Geometry check sheet. Reference: the model listing, model coordinates, mm. A direction names the side the tool comes from. Round coordinates to 2 decimals unless told otherwise and drop trailing zeros. Write each loop counter-clockwise with the first axis right and the second up, starting at its lowest first coordinate (ties: lowest second). Pieces come first, ordered by that corner, then holes.
Item 1: Cross-section at C-C (x = 24). Enter the section's corners in (y, z), then the cut area to 3 significant figures.
Item 2: Cross-section at B-B (y = 42). Enter the section's corners in (x, z).
Item 3: Access from +Z, -Z, +X, -X, +Y, -Y to the whole of each face (thin tool, end or side, straight path). Record for faces 1 (the face through (2, 8, 9.44)), 2 (the face through (6.27, 1.163, 4.689)), 3 (the face through (-0.5, 41, 4)), 4 (the face through (-0.5, 33, 10)).
Item 4: Cross-section at A-A (z = 8.75). Enter the section's corners in (x, y).
Item 5: Draft check along Y on faces 5 (the face through (6.27, 51.3, 4.63)), 6 (the face through (38.4, 26, 4)), 7 (the face through (18.04, 3.65, 1.27)), 8 (the face through (-1.57, 4.15, 0.11)). Enter one of: pulls with the +Y half, pulls with the -Y half, needs draft (parallel to the pull), parting line crosses it, or undercut.
Item 6: Cross-section at D-D (x = 34). Enter the section's corners in (y, z), then the cut area to 3 significant figures.
Item 7: Scan lines: probe 1 along Y at (x, z) = (16, 3); probe 2 along X at (y, z) = (20, 2.5); probe 3 along X at (y, z) = (44.5, 5.5). Record each from-to range of solid material in increasing order.
Item 8: Depth check by flat-ended pin: P1, Ø8, axis at x = 30.5, y = 36.5, coming from the -Z side; P2, Ø2, axis at x = 28, z = 4.5, coming from the +Y side; P3, Ø0.8, axis at y = 32, z = 11, coming from the +X side; P4, Ø1, axis at x = 2, y = 45, coming from the +Z side. Enter the tip coordinate at first touch or a pass-through.
from build123d import *

# Parameters (mm, degrees)
SKETCH003_R     = 0.75
PAD002_DEPTH    = 40.4
SKETCH002_W     = 37.4
SKETCH002_H     = 43
POCKET_DEPTH    = 13
SKETCH004_W     = 9
SKETCH004_H     = 3.2
POCKET001_DEPTH = 2
POCKET005_DEPTH = 2
POCKET006_DEPTH = 2
SKETCH015_W     = 46
SKETCH015_H     = 40.4
POCKET010_DEPTH = 2.5
SKETCH018_W     = 3.6
SKETCH018_H     = 1.8
SKETCH018_W_2   = 10
SKETCH018_W_3   = 3
PAD004_DEPTH    = 10.5
SKETCH020_W     = 38.2
SKETCH020_H     = 33.9
POCKET013_DEPTH = 2.6
POCKET015_DEPTH = 23.5
FILLET004_R     = 1.5
FILLET005_R     = 0.6
FILLET006_R     = 1.35


with BuildPart() as part:
    # Sketch003 → Pad002 (new body)
    with BuildSketch(Plane(origin=(-2, 0, 0), x_dir=(0, -1, 0), z_dir=(-1, 0, 0))):
        with BuildLine():
            Line((-3.2, 6), (1.170226, 1.888902))
            ThreePointArc((-2.940872, -2.481324), (1.29979, -2.35176), (1.170226, 1.888902))
            Line((-5.578597, 0), (-2.940872, -2.481324))
            Line((-5.578597, 0), (-46.821403, 0))
            Line((-46.821403, 0), (-49.459128, -2.481324))
            ThreePointArc((-53.570226, 1.888902), (-53.69979, -2.35176), (-49.459128, -2.481324))
            Line((-49.2, 6), (-53.570226, 1.888902))
            Line((-49.2, 9), (-49.2, 6))
            Line((-3.2, 9), (-49.2, 9))
            Line((-3.2, 9), (-3.2, 6))
        make_face()
        with Locations((-51.514677, -0.296211)):
            Circle(SKETCH003_R, mode=Mode.SUBTRACT)
        with Locations((-0.885323, -0.296211)):
            Circle(SKETCH003_R, mode=Mode.SUBTRACT)
    extrude(amount=-PAD002_DEPTH)

    # Sketch002 → Pocket (cut)
    with BuildSketch(Plane(origin=(0, 0, 0.7), x_dir=(-1, 0, 0), z_dir=(0, 0, -1))):
        with Locations((-18.2, 26.2)):
            Rectangle(SKETCH002_W, SKETCH002_H)
    extrude(amount=-POCKET_DEPTH, mode=Mode.SUBTRACT)

    # Sketch004 (on Face4 of Pocket) → Pocket001 (cut)
    with BuildSketch(Plane(origin=(-2, 0, 0), x_dir=(0, -1, 0), z_dir=(-1, 0, 0))):
        with Locations((-26.4, 5.93)):
            Rectangle(SKETCH004_W, SKETCH004_H)
    extrude(amount=-POCKET001_DEPTH, mode=Mode.SUBTRACT)

    # Sketch010 (on Face5 of Pocket001) → Pocket005 (cut)
    with BuildSketch(Plane.YZ.offset(38.4)):
        with BuildLine():
            ThreePointArc((7.8, 9.05), (6.4, 7.65), (7.8, 6.25))
            Line((7.8, 6.25), (12.8, 6.25))
            ThreePointArc((12.8, 6.25), (14.2, 7.65), (12.8, 9.05))
            Line((12.8, 9.05), (7.8, 9.05))
        make_face()
        with BuildLine():
            ThreePointArc((39.6, 9.05), (38.2, 7.65), (39.6, 6.25))
            Line((39.6, 6.25), (44.6, 6.25))
            ThreePointArc((44.6, 6.25), (46, 7.65), (44.6, 9.05))
            Line((44.6, 9.05), (39.6, 9.05))
        make_face()
    extrude(amount=-POCKET005_DEPTH, mode=Mode.SUBTRACT)

    # Sketch011 (on Face4 of Pocket005) → Pocket006 (cut)
    with BuildSketch(Plane(origin=(-2, 0, 0), x_dir=(0, -1, 0), z_dir=(-1, 0, 0))):
        with BuildLine():
            ThreePointArc((-44.6, 9.05), (-46, 7.65), (-44.6, 6.25))
            Line((-44.6, 6.25), (-39.6, 6.25))
            ThreePointArc((-39.6, 6.25), (-38.2, 7.65), (-39.6, 9.05))
            Line((-39.6, 9.05), (-44.6, 9.05))
        make_face()
        with BuildLine():
            ThreePointArc((-12.8, 9.05), (-14.2, 7.65), (-12.8, 6.25))
            Line((-12.8, 6.25), (-7.8, 6.25))
            ThreePointArc((-7.8, 6.25), (-6.4, 7.65), (-7.8, 9.05))
            Line((-7.8, 9.05), (-12.8, 9.05))
        make_face()
    extrude(amount=-POCKET006_DEPTH, mode=Mode.SUBTRACT)

    # Sketch015 (on Face2 of Pocket006) → Pocket010 (cut)
    with BuildSketch(Plane(origin=(0, 0, 9), x_dir=(0, -1, 0), z_dir=(0, 0, 1))):
        with Locations((-26.2, 18.2)):
            Rectangle(SKETCH015_W, SKETCH015_H)
    extrude(amount=-POCKET010_DEPTH, mode=Mode.SUBTRACT)

    # Sketch018 (on Face23 of Pocket001) → Pad004 (join)
    with BuildSketch(Plane(origin=(0, 0, 0.7), x_dir=(0, -1, 0), z_dir=(0, 0, 1))):
        with Locations((-45.9, 2.2)):
            Rectangle(SKETCH018_W, SKETCH018_H)
        with Locations((-6.5, 2.2)):
            Rectangle(SKETCH018_W, SKETCH018_H)
        with Locations((-6.5, 34.2)):
            Rectangle(SKETCH018_W, SKETCH018_H)
        with Locations((-45.9, 34.2)):
            Rectangle(SKETCH018_W, SKETCH018_H)
        with Locations((-26.2, 36)):
            Rectangle(SKETCH018_W_2, SKETCH018_H)
        with Locations((-20.3, 0.4)):
            Rectangle(SKETCH018_W_3, SKETCH018_H)
        with Locations((-32.5, 0.4)):
            Rectangle(SKETCH018_W_3, SKETCH018_H)
    extrude(amount=PAD004_DEPTH)

    # Sketch020 (on Face72 of Pad004) → Pocket013 (cut)
    with BuildSketch(Plane(origin=(0, 0, 11.2), x_dir=(0, -1, 0), z_dir=(0, 0, 1))):
        with Locations((-26.2, 18.2)):
            Rectangle(SKETCH020_W, SKETCH020_H)
    extrude(amount=-POCKET013_DEPTH, mode=Mode.SUBTRACT)

    # Sketch021 (on Face4 of Pocket010) → Pocket015 (cut)
    with BuildSketch(Plane.YZ.offset(29.95)):
        Polygon((3.2, 6), (3.2, 0), (5.8, 0), (5.8, -5.6), (-3.95, -5.6), (-3.95, 6), align=None)
        Polygon((49.2, 6), (49.2, 0), (46.6, 0), (46.6, -6.2), (57, -6.2), (57, 6), align=None)
    extrude(amount=-POCKET015_DEPTH, mode=Mode.SUBTRACT)

    # Fillet004
    fillet004_edges = [part.edges().sort_by_distance(p)[0] for p in [
        (18.2, 3.2, 0),
        (18.2, 49.2, 0),
        (-2, 26.2, 0),
        (-2, 4.259735, -1.240662),
        (-2, -1.29979, -2.35176),
        (-2, 1.014887, 3.944451),
        (38.4, 1.014887, 3.944451),
        (38.4, -1.29979, -2.35176),
        (38.4, 4.259735, -1.240662),
        (38.4, 26.2, 0),
        (38.4, 48.140265, -1.240662),
        (38.4, 53.69979, -2.35176),
        (38.4, 51.385113, 3.944451),
        (-2, 48.140265, -1.240662),
        (-2, 53.69979, -2.35176),
        (-2, 51.385113, 3.944451),
    ]]
    fillet(fillet004_edges, radius=FILLET004_R)

    # Fillet005
    fillet005_edges = [part.edges().sort_by_distance(p)[0] for p in [
        (6.45, 51.385113, 3.944451),
        (6.45, 53.69979, -2.35176),
        (6.45, 48.140265, -1.240662),
        (29.95, 51.385113, 3.944451),
        (29.95, 53.69979, -2.35176),
        (29.95, 48.140265, -1.240662),
        (29.95, 1.014887, 3.944451),
        (29.95, -1.29979, -2.35176),
        (29.95, 4.259735, -1.240662),
        (6.45, 1.014887, 3.944451),
        (6.45, -1.29979, -2.35176),
        (6.45, 4.259735, -1.240662),
    ]]
    fillet(fillet005_edges, radius=FILLET005_R)

    # Fillet006
    fillet006_edges = [part.edges().sort_by_distance(p)[0] for p in [
        (-1.25, 21.9, 4.33),
        (-1.25, 30.9, 4.33),
    ]]
    fillet(fillet006_edges, radius=FILLET006_R)


with BuildPart() as part_1:
    # Body002 placement: moved
    add(part.part.moved(Location((0, 0, 0.84))))


solid = part_1.part
Resolved:
1. outline: (3.2, 2.34) arc R1.5 ccw to (4.7, 0.84) - (47.7, 0.84) arc R1.5 ccw to (49.2, 2.34) - (49.2, 7.34) - (47.7, 7.34) - (47.7, 1.54) - (4.7, 1.54) - (4.7, 7.34) - (3.2, 7.34) - close
1. area: 48.6 mm2
2. outline: (-2, 2.34) arc R1.5 ccw to (-0.5, 0.84) - (36.9, 0.84) arc R1.5 ccw to (38.4, 2.34) - (38.4, 7.09) - (36.9, 7.09) - (36.9, 1.54) - (-0.5, 1.54) - (-0.5, 7.09) - (-2, 7.09) - close
3. face 1: +Z, +X, -X
3. face 2: +Z, -Y
3. face 3: +Z
3. face 4: +Z, -X, +Y, -Y
4. outline: (-0.5, 18.8) - (1.3, 18.8) - (1.3, 21.8) - (-0.5, 21.8) - close; (-0.5, 31) - (1.3, 31) - (1.3, 34) - (-0.5, 34) - close; (1.3, 4.7) - (3.1, 4.7) - (3.1, 8.3) - (1.3, 8.3) - close; (1.3, 44.1) - (3.1, 44.1) - (3.1, 47.7) - (1.3, 47.7) - close; (33.3, 4.7) - (35.1, 4.7) - (35.1, 8.3) - (33.3, 8.3) - close; (33.3, 44.1) - (35.1, 44.1) - (35.1, 47.7) - (33.3, 47.7) - close; (35.1, 21.2) - (36.9, 21.2) - (36.9, 31.2) - (35.1, 31.2) - close
5. face 5: pulls with the +Y half
5. face 6: needs draft
5. face 7: pulls with the -Y half
5. face 8: undercut
6. outline: (-1.17, 2.73) arc R3 ccw to (2.94, -1.64) - (5.58, 0.84) - (46.82, 0.84) - (49.46, -1.64) arc R3 ccw to (53.57, 2.73) - (49.2, 6.84) - (49.2, 7.34) - (47.7, 7.34) - (47.7, 12.04) - (45.3, 12.04) - (45.3, 9.44) - (44.1, 9.44) - (44.1, 1.54) - (8.3, 1.54) - (8.3, 9.44) - (7.1, 9.44) - (7.1, 12.04) - (4.7, 12.04) - (4.7, 7.34) - (3.2, 7.34) - (3.2, 6.84) - close; hole circle Ø1.5 at (0.89, 0.54); hole circle Ø1.5 at (51.51, 0.54)
6. area: 187 mm2
7. probe 1: y = 3.2 to 4.7, 47.7 to 49.2
7. probe 2: x = -2 to 1.3, 36.9 to 38.4
7. probe 3: x = -2 to -0.5, 1.3 to 3.1, 33.3 to 35.1, 36.9 to 38.4
8. P1: stops at z = 0.84
8. P2: stops at y = 49.2
8. P3: stops at x = 1.25
8. P4: stops at z = 12.04
